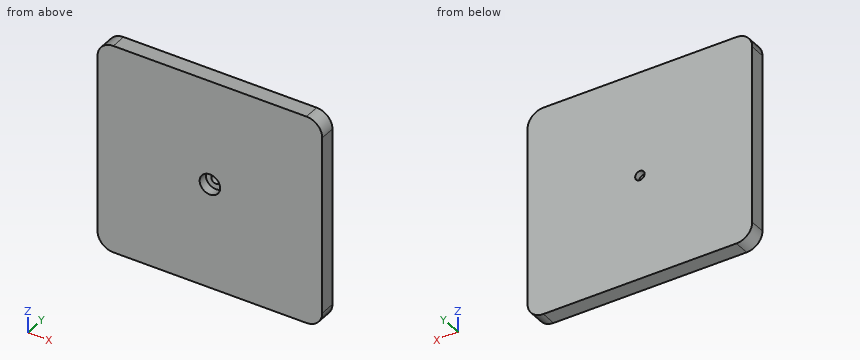
```python
from build123d import *

# Parameters (mm, degrees)
F0_W           = 71.148194
F0_H           = 66.397064
F1_DEPTH       = 5
F3_D           = 3
F3_CBORE_D     = 6.5
F3_CBORE_DEPTH = 3
F4_R           = 5


with BuildPart() as f1:
    # F0 (on Front) → F1 (new body)
    with BuildSketch(Plane.XZ):
        Rectangle(F0_W, F0_H)
    extrude(amount=F1_DEPTH)

    # F3 (through all)
    with Locations(Plane.XZ.offset(5)):
        with Locations((0, 0)):
            CounterBoreHole(F3_D / 2, F3_CBORE_D / 2, F3_CBORE_DEPTH)

    # F4
    f4_edges = [f1.edges().sort_by_distance(p)[0] for p in [
        (35.574097, -2.5, 33.198532),
        (-35.574097, -2.5, 33.198532),
        (35.574097, -2.5, -33.198532),
        (-35.574097, -2.5, -33.198532),
    ]]
    fillet(f4_edges, radius=F4_R)


solid = f1.part
```
Work out the finished part from the listing and answer in its coordinate system (mm). Give positions to 0.01 mm unless a question says otherwise; leave off trailing zeros. Write each loop counter-clockwise with the first axis right and the second up, starting at its lowest first coordinate (ties: lowest second). Pieces come first, ordered by that corner, then holes.
(1) The part is cut by section B-B on z = 0. Write down the section's boundary in (x, y).
Final values:
outline: (-35.57, -5) - (-3.25, -5) - (-3.25, -2) - (-1.5, -2) - (-1.5, 0) - (-35.57, 0) - close; (1.5, -2) - (3.25, -2) - (3.25, -5) - (35.57, -5) - (35.57, 0) - (1.5, 0) - close
(2) Straight lines are drawn through the part: line 1 (Z direction, x = 0, y = -2.85); line 2 (Z direction, x = 0, y = -0.9); line 3 (X direction, y = -4.25, z = 30). For each, find the intervals that lie inside material, in ascending order.
Final values:
line 1: z = -33.2 to -3.25, 3.25 to 33.2
line 2: z = -33.2 to -1.5, 1.5 to 33.2
line 3: x = -35.24 to 35.24
(3) The part is cut by section A-A on x = 0. Write down the section's boundary in (y, z).
Final values:
outline: (-5, -33.2) - (0, -33.2) - (0, -1.5) - (-2, -1.5) - (-2, -3.25) - (-5, -3.25) - close; (-5, 3.25) - (-2, 3.25) - (-2, 1.5) - (0, 1.5) - (0, 33.2) - (-5, 33.2) - close
(4) A flat-ended cylindrical pin translates along its axis: pin 1 Ø3 at (x, z) = (-1, -1) entering from -Y. Find the tip coordinate at first contact, or state that the pin passes through.
Final values:
pin 1: stops at y = -2
